CAD build for the part. Positions are in the model's coordinates, mm. A direction names the side the tool comes from. Give positions to 0.01 mm unless a question says otherwise; leave off trailing zeros. Order: outer loops, then holes, each group sorted by start corner. A loop starts at its lowest first (then second) coordinate and runs counter-clockwise, first axis right, second up.
from build123d import *

# Parameters (mm, degrees)
SKETCH_1_W          = 90
SKETCH_1_H          = 150
EXTRUDE_1_DEPTH     = 80
SKETCH_2_R          = 13
CUT_EXTRUDE_1_DEPTH = 3
SKETCH_3_R          = 4
CUT_EXTRUDE_2_DEPTH = 10
SKETCH_4_R          = 4
CUT_EXTRUDE_3_DEPTH = 7


with BuildPart() as part:
    # 草图1 → 凸台-拉伸1 (new body)
    with BuildSketch(Plane.XY):
        Rectangle(SKETCH_1_W, SKETCH_1_H)
    extrude(amount=EXTRUDE_1_DEPTH)

    # 草图2 → 切除-拉伸1 (cut)
    with BuildSketch(Plane.XY.offset(80)):
        with Locations((18, -18)):
            Circle(SKETCH_2_R)
        with Locations((-18, 18)):
            Circle(SKETCH_2_R)
    extrude(amount=-CUT_EXTRUDE_1_DEPTH, mode=Mode.SUBTRACT)

    # 草图3 → 切除-拉伸2 (cut)
    with BuildSketch(Plane.XY.offset(80)):
        with Locations((2, 18)):
            Circle(SKETCH_3_R)
        with Locations((-38, 18)):
            Circle(SKETCH_3_R)
        with Locations((-2, -18)):
            Circle(SKETCH_3_R)
        with Locations((38, -18)):
            Circle(SKETCH_3_R)
    extrude(amount=-CUT_EXTRUDE_2_DEPTH, mode=Mode.SUBTRACT)

    # 草图4 → 切除-拉伸3 (cut)
    with BuildSketch(Plane(origin=(0, 0, 0), x_dir=(-1, 0, 0), z_dir=(0, 0, -1))):
        with Locations((-19.5, 60.372983346)):
            Circle(SKETCH_4_R)
        with Locations((-19.5, -34.627016654)):
            Circle(SKETCH_4_R)
        with Locations((19.5, -34.627016654)):
            Circle(SKETCH_4_R)
        with Locations((-19.5, 34.627016654)):
            Circle(SKETCH_4_R)
        with Locations((-19.5, -60.372983346)):
            Circle(SKETCH_4_R)
        with Locations((19.5, -60.372983346)):
            Circle(SKETCH_4_R)
        with Locations((19.5, 34.627016654)):
            Circle(SKETCH_4_R)
        with Locations((19.5, 60.372983346)):
            Circle(SKETCH_4_R)
    extrude(amount=-CUT_EXTRUDE_3_DEPTH, mode=Mode.SUBTRACT)


solid = part.part
1. Wall check: line 1 (Y direction, x = -19, z = 4); line 2 (Y direction, x = 19.5, z = 4.75); line 3 (Y direction, x = -18, z = 78.45). Give the ranges that are in metal, low to high.
2. 3-axis set-ups, long thin cutter, end or side, ignore diameter. For faces 1 (the flat face through (45, -1, 39)), 2 (the flat face through (-38, 18, 70)), 3 (the flat face through (-19, 35, 7)): which of +Z, -Z, +X, -X, +Y, -Y reach the whole face in a straight line?
3. Saw through at B-B on x = -18. Give the cut face in (y, z), plus the area to 3 significant figures.
4. Saw through at A-A on y = -18. Give the cut face in (x, z), plus the area to 3 significant figures.
5. Pin check, flat tips, straight feed: P1, Ø5, axis at x = 19.5, y = 60.37, coming from the -Z side; P2, Ø4, axis at x = 1, y = 18, coming from the +Z side. Stop position of each tip, or through.
Reported:
1. line 1: y = -75 to -64.34, -56.4 to -38.6, -30.66 to 30.66, 38.6 to 56.4, 64.34 to 75
1. line 2: y = -75 to -64.37, -56.37 to -38.63, -30.63 to 30.63, 38.63 to 56.37, 64.37 to 75
1. line 3: y = -75 to 5, 31 to 75
2. face 1: +Z, -Z, +X, +Y, -Y
2. face 2: +Z
2. face 3: -Z
3. outline: (-75, 0) - (-64.08, 0) - (-64.08, 7) - (-56.66, 7) - (-56.66, 0) - (-38.34, 0) - (-38.34, 7) - (-30.92, 7) - (-30.92, 0) - (30.92, 0) - (30.92, 7) - (38.34, 7) - (38.34, 0) - (56.66, 0) - (56.66, 7) - (64.08, 7) - (64.08, 0) - (75, 0) - (75, 80) - (31, 80) - (31, 77) - (5, 77) - (5, 80) - (-75, 80) - close
3. area: 11,700 mm2
4. outline: (-45, 0) - (45, 0) - (45, 80) - (42, 80) - (42, 70) - (34, 70) - (34, 80) - (31, 80) - (31, 77) - (5, 77) - (5, 80) - (2, 80) - (2, 70) - (-6, 70) - (-6, 80) - (-45, 80) - close
4. area: 6,960 mm2
5. P1: stops at z = 7
5. P2: stops at z = 70
